Input: part model. Units: mm. Frame: model coordinates. Coordinates: 2 decimals unless noted, no trailing zeros. Order: outer loops, then holes, each group sorted by start corner. A loop starts at its lowest first (then second) coordinate and runs counter-clockwise, first axis right, second up. Notation, with made-up numbers: M 18.25,45.25 L 41.25,45.25 A6 ccw 41.25,54.25 Z; hole C 83.5,-38 d4. An arc over 180 degrees is marked long. One line per item, written item: value.
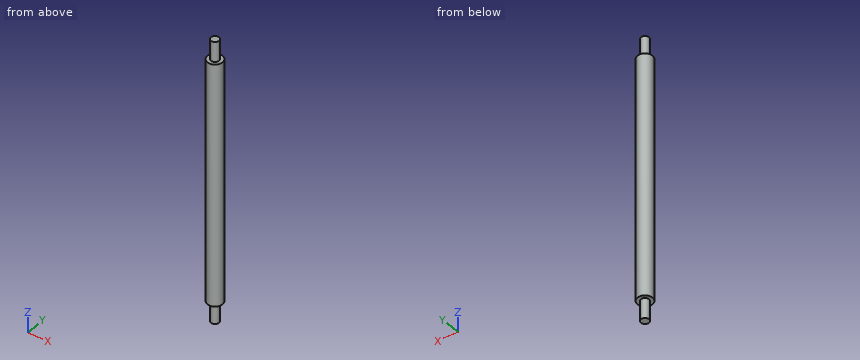
```python
from build123d import *

# Parameters (mm, degrees)
SKETCH1_R           = 7.5
BOSS_EXTRUDE1_DEPTH = 242
SKETCH2_R           = 4
BOSS_EXTRUDE2_DEPTH = 20


with BuildPart() as part:
    # Sketch1 → Boss-Extrude1 (new body)
    with BuildSketch(Plane.XY):
        Circle(SKETCH1_R)
    extrude(amount=BOSS_EXTRUDE1_DEPTH)

    # Sketch2 → Boss-Extrude2 (add)
    with BuildSketch(Plane.XY.offset(242)):
        Circle(SKETCH2_R)
    boss_extrude2 = extrude(amount=BOSS_EXTRUDE2_DEPTH)

    # Mirror1: Boss-Extrude2 across plane
    add(boss_extrude2.mirror(Plane.XY.offset(121)))


solid = part.part
```
(1) Cut plane C-C on z = 238. Output: boundary loops of the cut face in (x, y).
Data:
outline: C 0,0 d15
(2) Ray query, line 1 (Z direction, x = -3.5, y = 2); line 2 (Y direction, x = -0.25, z = 63); line 3 (Y direction, x = 1, z = 164.5). Return the intervals inside material, ascending. Write a range as from..to.
Data:
line 1: z = 0..242
line 2: y = -7.5..7.5
line 3: y = -7.43..7.43
(3) Cut plane A-A on x = 0. Output: boundary loops of the cut face in (y, z).
Data:
outline: M -7.5,0 L -4,0 L -4,-20 L 4,-20 L 4,0 L 7.5,0 L 7.5,242 L 4,242 L 4,262 L -4,262 L -4,242 L -7.5,242 Z
(4) First-contact query: pin 1 (5 mm diameter, centred on y = 4, z = 146.5, fed in from +X); pin 2 (1 mm diameter, centred on x = -4, y = -5.5, fed in from -Z); pin 3 (2 mm diameter, centred on y = -1.5, z = 134, fed in from -X). Flat tips, straight axial feed; report the tip coordinate or a pass-through.
Data:
pin 1: stops at x = 7.35
pin 2: stops at z = 0
pin 3: stops at x = -7.48
